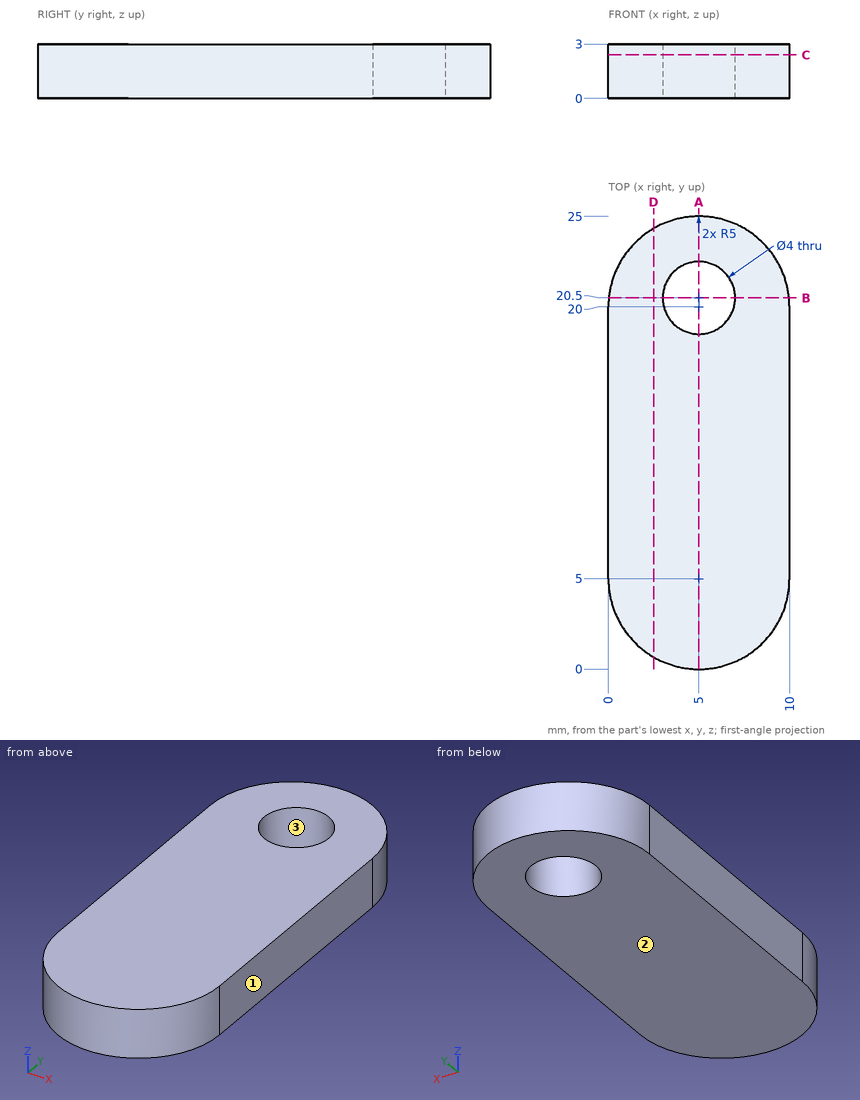
Design review of the part shown in the three views and the two pictorial views. Dimensions are in mm from the part's minimum x, y and z. Round coordinates to 2 decimals unless told otherwise and drop trailing zeros. Order: outer loops, then holes, each group sorted by start corner. A loop starts at its lowest first (then second) coordinate and runs counter-clockwise, first axis right, second up.
Item 1: Draft analysis for pull direction X (two halves, no side actions). For the marked faces 1, 2 and 3, state which applies: released by +X, released by -X, zero draft, split by the parting line, or undercut.
Working result:
face 1: released by +X
face 2: zero draft
face 3: undercut
Item 2: Add section A-A, the plane x = 5. State the section outline as (y, z) points.
Working result:
outline: (0, 0) - (18.5, 0) - (18.5, 3) - (0, 3) - close; (22.5, 0) - (25, 0) - (25, 3) - (22.5, 3) - close
Item 3: Add section C-C, the plane z = 2.4. State the section outline as (x, y) points.
Working result:
outline: (0, 5) arc R5 ccw to (10, 5) - (10, 20) arc R5 ccw to (0, 20) - close; hole circle Ø4 at (5, 20.5)
Item 4: Add section D-D, the plane x = 2.5. State the section outline as (y, z) points, and give its area (3 significant figures).
Working result:
outline: (0.67, 0) - (24.33, 0) - (24.33, 3) - (0.67, 3) - close
area: 71.0 mm2
Item 5: Add section B-B, the plane y = 20.5. State the section outline as (x, z) points, and give its area (3 significant figures).
Working result:
outline: (0.03, 0) - (3, 0) - (3, 3) - (0.03, 3) - close; (7, 0) - (9.97, 0) - (9.97, 3) - (7, 3) - close
area: 17.8 mm2
Item 6: To check wall thickness, follow probe 1 along Y at (x, z) = (5, 1.85); probe 2 along X at (y, z) = (18.75, 1.35); probe 3 along Y at (x, z) = (6.5, 0.85). State the ranges of each line that lie inside material, in increasing order.
Working result:
probe 1: y = 0 to 18.5, 22.5 to 25
probe 2: x = 0 to 4.03, 5.97 to 10
probe 3: y = 0.23 to 19.18, 21.82 to 24.77
Item 7: For pin 1 (1 mm diameter, centred on x = 3.5, z = 1.5, fed in from +Y), flat-tipped, find the tip position at first contact; note if it passes through.
Working result:
pin 1: stops at y = 24.9
